Here's the drawing with two shaded views (mm, measured from the low corner). I have some questions. A direction names the side the tool comes from. Give positions to 0.01 mm unless a question says otherwise; leave off trailing zeros. Loops run counter-clockwise (first coordinate to the right, second up) from the corner with the lowest first, then second, coordinate; pieces in that order, holes last. Notation, with made-up numbers: (-2, -26.75) - (47, -26.75) arc R22 cw to (47, -7.75) - close; hole circle Ø2 at (-28, 12.25). An arc over 180 degrees is marked (long way). Answer as a JSON object with one key per item and string values. Group by question number.
Item 1: Will these pins go through, and if not, where does the flat tip stop? pin 1 (8.5 mm diameter, centred on x = 6.35, z = 6.35, fed in from +Y) (3 decimals); pin 2 (4 mm diameter, centred on x = 31.75, z = 6.35, fed in from -Y); pin 3 (1 mm diameter, centred on x = 25.5, y = 5.5, fed in from -Z).
Item 2: Suppose I cut it at C-C on y = 1.5. Write out the boundary of the cut face in (x, z), and give its area (3 significant figures).
Item 3: Suppose I cut it at A-A on x = 6.35. Count the separate pieces of the cut face and the enclosed holes in it, and give its area (3 significant figures).
Item 4: Which directions (+Z, -Z, +X, -X, +Y, -Y) give clear straight access to the entire face, cutting with the end or side of a thin tool? Please do the marked faces 1 and 2.
Item 5: Please list where these lines run through material, in increasing order: L1, parallel to X at y = 0.85, z = 31.75; L2, parallel to Z at x = 31.75, y = 2.75; L3, parallel to Z at x = 31, y = 3 (1 decimal).
Item 6: Suppose I cut it at B-B on z = 6.35. Write out the boundary of the cut face in (x, y) (1 decimal).
Item 7: Suppose I cut it at D-D on y = 4.25. Write out the boundary of the cut face in (x, z), and give its area (3 significant figures).
Item 8: Thinking about a two-plate mould opening in Z: for the marked faces 3 and 4, which applies, pulls with the +Z half, pulls with the -Z half, needs draft (parallel to the pull), parting line crosses it, or undercut?
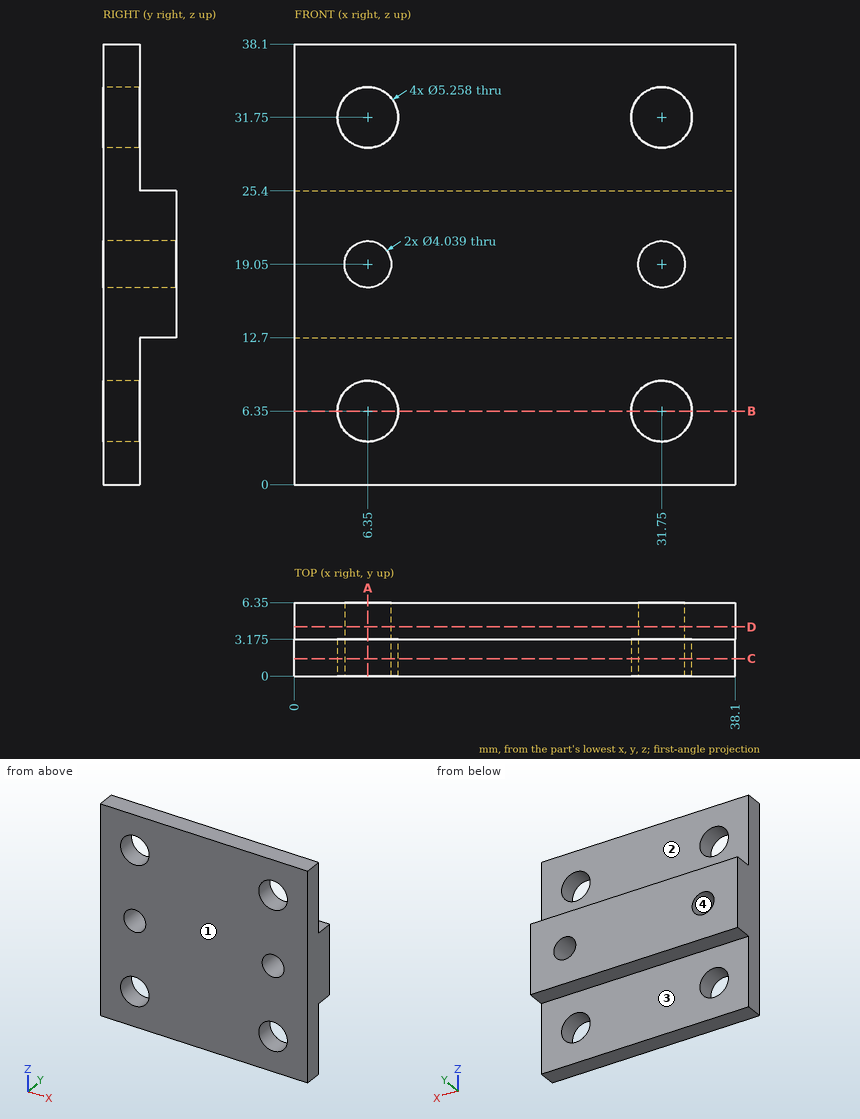
Worked out:
{
 "1": {"pin 1": "stops at y = 3.175", "pin 2": "passes through", "pin 3": "stops at z = 12.7"},
 "2": {"outline": "(0, 0) - (38.1, 0) - (38.1, 38.1) - (0, 38.1) - close; hole circle Ø5.26 at (6.35, 6.35); hole circle Ø5.26 at (6.35, 31.75); hole circle Ø4.04 at (6.35, 19.05); hole circle Ø5.26 at (31.75, 6.35); hole circle Ø5.26 at (31.75, 31.75); hole circle Ø4.04 at (31.75, 19.05)", "area": "1,340 mm2"},
 "3": {"separate pieces": "4", "enclosed holes": "0", "area": "102 mm2"},
 "4": {"face 1": "+Z, -Z, +X, -X, -Y", "face 2": "+Z, +X, -X, +Y"},
 "5": {"L1": "x = 0 to 3.72, 8.98 to 29.12, 34.38 to 38.1", "L2": "z = 0 to 3.72, 8.98 to 17.03, 21.07 to 29.12, 34.38 to 38.1", "L3": "z = 0 to 3.8, 8.9 to 17.2, 20.9 to 29.2, 34.3 to 38.1"},
 "6": {"outline": "(0, 0) - (3.7, 0) - (3.7, 3.2) - (0, 3.2) - close; (9, 0) - (29.1, 0) - (29.1, 3.2) - (9, 3.2) - close; (34.4, 0) - (38.1, 0) - (38.1, 3.2) - (34.4, 3.2) - close"},
 "7": {"outline": "(0, 12.7) - (38.1, 12.7) - (38.1, 25.4) - (0, 25.4) - close; hole circle Ø4.04 at (6.35, 19.05); hole circle Ø4.04 at (31.75, 19.05)", "area": "458 mm2"},
 "8": {"face 3": "needs draft", "face 4": "undercut"}
}
